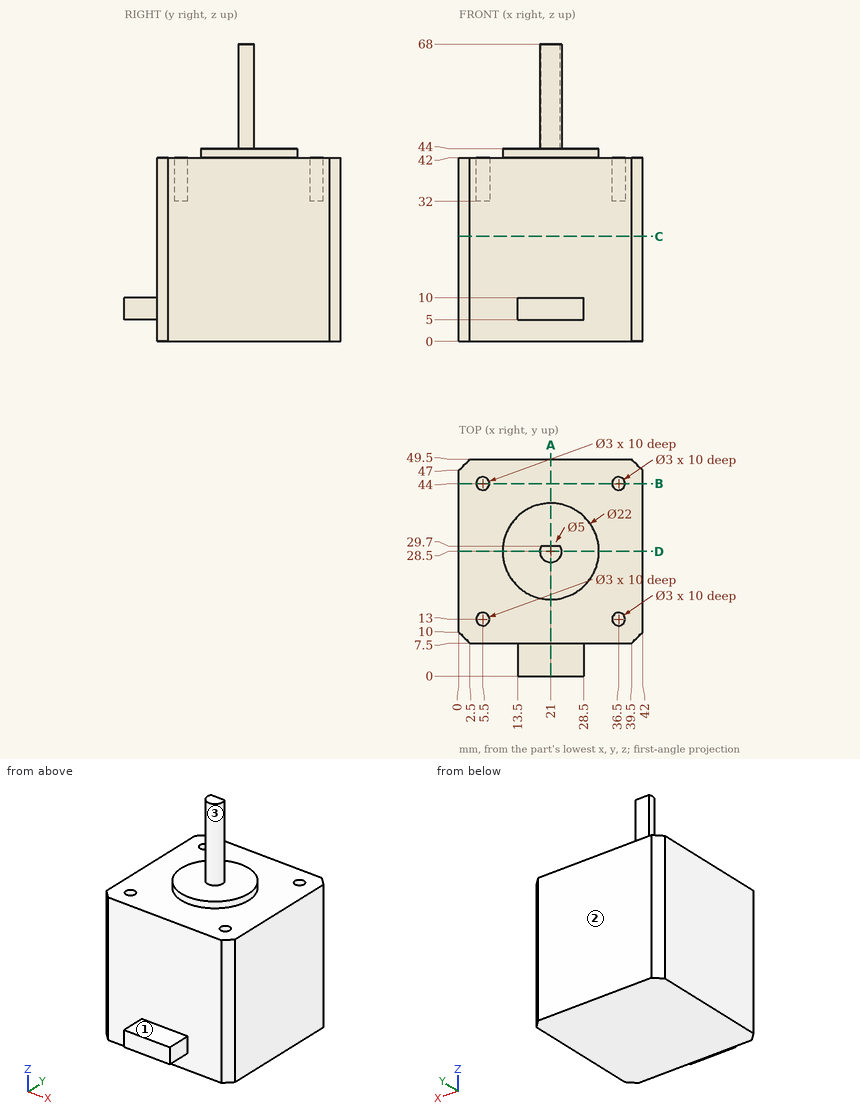
Verification items for this drawing (mm, ordinates from the low corner). A direction names the side the tool comes from. Coordinates: 2 decimals unless noted, no trailing zeros. Order: outer loops, then holes, each group sorted by start corner. A loop starts at its lowest first (then second) coordinate and runs counter-clockwise, first axis right, second up. Notation, with made-up numbers: M 28.5,-23.5 L 52.5,-23.5 A19 ccw 52.5,-13.5 Z; hole C 60,70.5 d4. An arc over 180 degrees is marked long. Answer as a JSON object with one key per item and string values.
Q1. Cross-section at D-D on y = 28.5. Record the cut outline in (x, z), and give its area (3 significant figures).
Results are:
{"outline": "M 0,0 L 42,0 L 42,42 L 32,42 L 32,44 L 23.5,44 L 23.5,68 L 18.5,68 L 18.5,44 L 10,44 L 10,42 L 0,42 Z", "area": "1,930 mm²"}
Q2. Cross-section at C-C on z = 24. Record the cut outline in (x, y).
Results are:
{"outline": "M 0,10 L 2.5,7.5 L 39.5,7.5 L 42,10 L 42,47 L 39.5,49.5 L 2.5,49.5 L 0,47 Z"}
Q3. Tool access check on the marked faces 1, 2 and 3. Record the directions out of +Z, -Z, +X, -X, +Y, -Y that give a thin tool (end or side, any length) a straight path to the whole face; none if there is none.
Results are:
{"face 1": "+Z, +X, -X, -Y", "face 2": "+Z, -Z, +X, -X, +Y", "face 3": "+Z"}
Q4. Cross-section at A-A on x = 21. Record the cut outline in (y, z).
Results are:
{"outline": "M 0,5 L 7.5,5 L 7.5,0 L 49.5,0 L 49.5,42 L 39.5,42 L 39.5,44 L 29.7,44 L 29.7,68 L 26,68 L 26,44 L 17.5,44 L 17.5,42 L 7.5,42 L 7.5,10 L 0,10 Z"}
Q5. Cross-section at B-B on y = 44. Record the cut outline in (x, z).
Results are:
{"outline": "M 0,0 L 42,0 L 42,42 L 38,42 L 38,32 L 35,32 L 35,42 L 7,42 L 7,32 L 4,32 L 4,42 L 0,42 Z"}
Q6. Depth check by flat-ended pin: pin 1 Ø1.5 at (x, y) = (37, 13) entering from +Z; pin 2 Ø2 at (y, z) = (21.5, 24.5) entering from -X; pin 3 Ø3.5 at (x, y) = (5.5, 13) entering from +Z; pin 4 Ø1.5 at (x, z) = (12.5, 16) entering from -Y. Enter the tip coordinate at first touch or a pass-through.
Results are:
{"pin 1": "stops at z = 32", "pin 2": "stops at x = 0", "pin 3": "stops at z = 42", "pin 4": "stops at y = 7.5"}
Q7. Scan lines: line 1 (Y direction, x = 5.5, z = 36.5); line 2 (Z direction, x = 6, y = 30); line 3 (Y direction, x = 30.5, z = 12.5). Record each from-to range of solid material in increasing order.
Results are:
{"line 1": "y = 7.5 to 11.5, 14.5 to 42.5, 45.5 to 49.5", "line 2": "z = 0 to 42", "line 3": "y = 7.5 to 49.5"}
